```python
from build123d import *

# Parameters (mm, degrees)
SKETCH1_R           = 25
BOSS_EXTRUDE1_DEPTH = 200
SKETCH9_R           = 30
BOSS_EXTRUDE4_DEPTH = 15


with BuildPart() as part:
    # Sketch1 → Boss-Extrude1 (new body)
    with BuildSketch(Plane(origin=(0, 0, 0), x_dir=(1, 0, 0), z_dir=(0, 1, 0))):
        Circle(SKETCH1_R)
    extrude(amount=BOSS_EXTRUDE1_DEPTH)

    # Sketch9 → Boss-Extrude4 (add, symmetric)
    with BuildSketch(Plane(origin=(0, 0, 0), x_dir=(0, 0, -1), z_dir=(1, 0, 0))):
        Circle(SKETCH9_R)
    extrude(amount=BOSS_EXTRUDE4_DEPTH, both=True)


solid = part.part
```
The model under review builds one solid part; all positions refer to its coordinate system, in mm. Round coordinates to 2 decimals unless told otherwise and drop trailing zeros. Write each loop counter-clockwise with the first axis right and the second up, starting at its lowest first coordinate (ties: lowest second). Pieces come first, ordered by that corner, then holes.
(1) Mouldability with a two-part tool opening along Y and no side actions: class faces 1 (the flat face through (0, 200, 0)), 2 (the flat face through (-19, 0, 0)), 3 (the cylindrical face through (-24.976, 98.6, -1.099)), 4 (the cylindrical face through (0.21, -29.983, 1.013)) as +Y half, -Y half, draft (parallel to the pull), parting line (faces both ways), or undercut.
(2) We need section B-B on y = 3.5. Give the boundary of the cut face in (x, z).
(3) We need section C-C on x = -3. Give the boundary of the cut face in (y, z).
(4) Insertion check: pin 1 (1 mm diameter, centred on x = 7.5, y = 128.5, fed in from -Z); pin 2 (6 mm diameter, centred on y = 49, z = 5, fed in from -X); pin 3 (5 mm diameter, centred on x = -19, z = -2, fed in from -Y). Each pin has a flat end and moves straight along its axis. Give the tip position at first contact, or say it passes through.
(5) We need section A-A on z = -17. Give the boundary of the cut face in (x, y), and give its area (3 significant figures).
(6) Wall thickness on L1, parallel to Y at x = 8.5, z = 1; L2, parallel to Z at x = 20, y = 190; L3, parallel to Y at x = -19.5, z = -9.5: over which ranges is each line inside the solid? List them lowest first.
(7) We need section D-D on x = -18. Give the boundary of the cut face in (y, z).
Findings below:
1. face 1: +Y half
1. face 2: -Y half
1. face 3: draft
1. face 4: parting line
2. outline: (-15, -29.8) - (15, -29.8) - (15, -20) arc R25 ccw to (15, 20) - (15, 29.8) - (-15, 29.8) - (-15, 20) arc R25 ccw to (-15, -20) - close
3. outline: (16.85, -24.82) - (200, -24.82) - (200, 24.82) - (16.85, 24.82) arc R30 ccw (long way) to start
4. pin 1: stops at z = -24
4. pin 2: stops at x = -24.92
4. pin 3: stops at y = 0
5. outline: (-18.33, 0) - (-15, 0) - (-15, -24.72) - (15, -24.72) - (15, 0) - (18.33, 0) - (18.33, 200) - (-18.33, 200) - close
5. area: 8,070 mm2
6. L1: y = -29.98 to 200
6. L2: z = -15 to 15
6. L3: y = 0 to 200
7. outline: (0, -17.35) - (200, -17.35) - (200, 17.35) - (0, 17.35) - close
